from build123d import *

# Parameters (mm, degrees)
F0_W     = 25.4
F0_H     = 25.4
F0_W_2   = 22.225
F0_H_2   = 22.225
F1_DEPTH = 50.8
F2_W     = 6.35
F2_H     = 38.1
F2_W_2   = 38.1
F2_H_2   = 6.35
F3_DEPTH = 19.05
F4_R     = 3.9751
F5_DEPTH = 25.4
F6_R     = 3.9751
F7_DEPTH = 25.4


with BuildPart() as f1:
    # F0 (on Front) → F1 (new body)
    with BuildSketch(Plane.XZ):
        with Locations((12.7, 12.7)):
            Rectangle(F0_W, F0_H)
        with Locations((12.7, 12.7)):
            Rectangle(F0_W_2, F0_H_2, mode=Mode.SUBTRACT)
    extrude(amount=F1_DEPTH)

    # F2 (on Front) → F3 (join)
    with BuildSketch(Plane.XZ):
        with Locations((12.7, -19.05)):
            Rectangle(F2_W, F2_H)
        with Locations((-19.05, 12.7)):
            Rectangle(F2_W_2, F2_H_2)
    extrude(amount=F3_DEPTH)

    # F4 (on face) → F5 (cut)
    with BuildSketch(Plane(origin=(9.525, 0, 0), x_dir=(0, -1, 0), z_dir=(-1, 0, 0))):
        with Locations((9.525, -25.4)):
            Circle(F4_R)
    extrude(amount=-F5_DEPTH, mode=Mode.SUBTRACT)

    # F6 (on face) → F7 (cut)
    with BuildSketch(Plane(origin=(0, 0, 9.525), x_dir=(1, 0, 0), z_dir=(0, 0, -1))):
        with Locations((-25.4, 9.525)):
            Circle(F6_R)
    extrude(amount=-F7_DEPTH, mode=Mode.SUBTRACT)


solid = f1.part
Could you check a few things on this model? Use its own coordinates, in mm. A direction names the side the tool comes from. Coordinates: 2 decimals unless noted, no trailing zeros. Order: outer loops, then holes, each group sorted by start corner. A loop starts at its lowest first (then second) coordinate and runs counter-clockwise, first axis right, second up. Notation, with made-up numbers: (56, 49.25) -> (93, 49.25) arc R12 ccw to (93, 66.25) -> close; hole circle Ø3 at (46.25, 27.5). An arc over 180 degrees is marked (long way). One line per question, with ' | ' between items.
Q1. If I drill on L1, parallel to X at y = -11.5, z = 21.5; L2, parallel to X at y = -1.5, z = 13, over which ranges is the centre line in solid material (lowest first)?
Return value:
L1: 0 to 1.59, 23.81 to 25.4 | L2: -38.1 to 1.59, 23.81 to 25.4
Q2. Thinking about a two-plate mould opening in X: for faces 6 (the face through (1.587, -25, 13)), 7 (the face through (13, -25, 0)), 8 (the face through (15.875, -9, -19)), 9 (the face through (13, -25, 1.587)), which applies, pulls with the +X half, pulls with the -X half, needs draft (parallel to the pull), parting line crosses it, or undercut?
Return value:
face 6: undercut | face 7: needs draft | face 8: pulls with the +X half | face 9: undercut
Q3. I'm going to push flat-ended pins straight in: P1, Ø18, axis at x = 8.5, y = -33, coming from the -Z side; P2, Ø21, axis at x = -22, y = -5.5, coming from the -Z side (3 decimals); P3, Ø2, axis at y = -14, z = -28, coming from the +X side (3 decimals); P4, Ø5, axis at y = -9.525, z = -25.4, coming from the -X side. Where does each tip first touch, or does it pass through?
Return value:
P1: z = 0 | P2: z = 9.525 | P3: x = 15.875 | P4: through
Q4. Imagine slicing it at B-B on z = -25.4. Please give me the cut outline in (x, y) (3 decimals).
Return value:
outline: (9.525, -19.05) -> (15.875, -19.05) -> (15.875, -13.5) -> (9.525, -13.5) -> close; (9.525, -5.55) -> (15.875, -5.55) -> (15.875, 0) -> (9.525, 0) -> close
Q5. Imagine slicing it at C-C on y = -3.5. Please give me the cut outline in (x, z) (1 decimal).
Return value:
outline: (-38.1, 9.5) -> (0, 9.5) -> (0, 0) -> (9.5, 0) -> (9.5, -38.1) -> (15.9, -38.1) -> (15.9, 0) -> (25.4, 0) -> (25.4, 25.4) -> (0, 25.4) -> (0, 15.9) -> (-38.1, 15.9) -> close; hole (1.6, 1.6) -> (23.8, 1.6) -> (23.8, 23.8) -> (1.6, 23.8) -> close
Q6. Imagine slicing it at D-D on z = 13. State how many separate pieces and enclosed holes the cut face has, and give its area (3 significant figures).
Return value:
separate pieces: 2 | enclosed holes: 1 | area: 837 mm²
Q7. Imagine slicing it at A-A on x = -25.4. Please give me the cut outline in (y, z) (3 decimals).
Return value:
outline: (-19.05, 9.525) -> (-13.5, 9.525) -> (-13.5, 15.875) -> (-19.05, 15.875) -> close; (-5.55, 9.525) -> (0, 9.525) -> (0, 15.875) -> (-5.55, 15.875) -> close
Q8. On a 3-axis mill with a long thin cutter (end or side, diameter ignored), from which of +Z, -Z, +X, -X, +Y, -Y can I reach the whole of each face in a straight line? I mean faces 1 (the face through (-19, -9, 15.875)), 2 (the face through (9.525, -9, -19)), 3 (the face through (23.812, -25, 13)), 4 (the face through (-29.37, -9.7, 12.66)), 5 (the face through (-38.1, -9, 13)). Say none if no direction works.
Return value:
face 1: +Z, -X, +Y, -Y | face 2: -Z, -X, +Y, -Y | face 3: +Y, -Y | face 4: +Z, -Z | face 5: +Z, -Z, -X, +Y, -Y
